Design review of the part shown in the three views and the two pictorial views. Dimensions are in mm from the part's minimum x, y and z. A direction names the side the tool comes from. Give positions to 0.01 mm unless a question says otherwise; leave off trailing zeros. Order: outer loops, then holes, each group sorted by start corner. A loop starts at its lowest first (then second) coordinate and runs counter-clockwise, first axis right, second up. Notation, with made-up numbers: (82, -36) - (113, -36) arc R13 cw to (113, -25) - close; hole circle Ø1 at (55.25, 84.25). An arc over 180 degrees is marked (long way). Put each result on its own line as item: value.
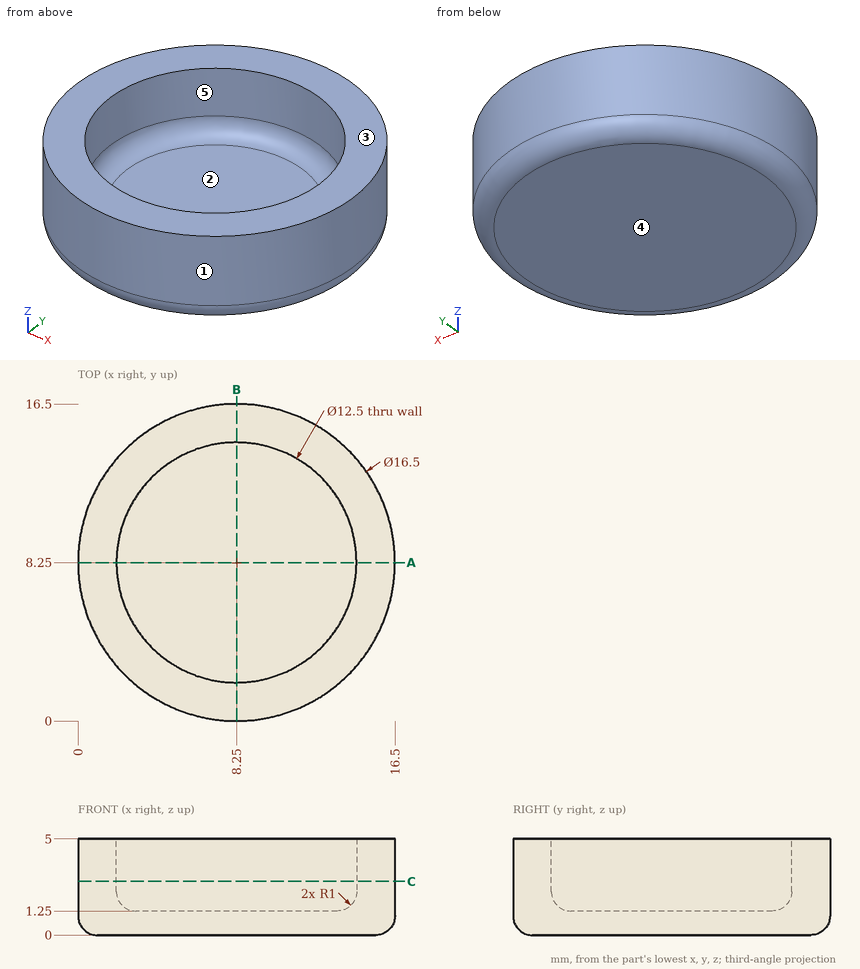
(1) The part is to be moulded in two halves that separate along Y. For the marked faces 1, 2 and 3, say which applies: pulls with the +Y half, pulls with the -Y half, needs draft (parallel to the pull), parting line crosses it, or undercut.
The answers:
face 1: parting line crosses it
face 2: undercut
face 3: needs draft
(2) For the marked faces 4 and 5, list the 3-axis set-ups (+Z, -Z, +X, -X, +Y, -Y) from which the entire face can be reached by the end or side of a thin tool; tool diameter is ignored.
The answers:
face 4: -Z, +X, -X, +Y, -Y
face 5: +Z
(3) Take a section at A-A, the plane y = 8.25. Write out the cut boundary in (x, z).
The answers:
outline: (0, 1) arc R1 ccw to (1, 0) - (15.5, 0) arc R1 ccw to (16.5, 1) - (16.5, 5) - (14.5, 5) - (14.5, 2.25) arc R1 cw to (13.5, 1.25) - (3, 1.25) arc R1 cw to (2, 2.25) - (2, 5) - (0, 5) - close
(4) Take a section at C-C, the plane z = 2.8. Write out the cut boundary in (x, y), then the cut area to 3 significant figures.
The answers:
outline: circle Ø16.5 at (8.25, 8.25); hole circle Ø12.5 at (8.25, 8.25)
area: 91.1 mm^2
(5) Clearance check with flat-ended pins moving along their axes: pin 1 Ø7.5 at (x, y) = (8.25, 8.25) entering from -Z; pin 2 Ø3 at (y, z) = (13, 3) entering from -X; pin 3 Ø1 at (x, y) = (8.5, 11) entering from +Z; pin 4 Ø1.5 at (y, z) = (2, 3) entering from -X. State where each tip first meets the part, or that it passes through.
The answers:
pin 1: z = 0
pin 2: x = 0.67
pin 3: z = 1.25
pin 4: x = 2.1
(6) Wall thickness on L1, parallel to Y at x = 8.25, z = 3.2; L2, parallel to X at y = 8.5, z = 2.3 (3 decimals); L3, parallel to Z at x = 8.75, y = 4.5: over which ranges is each line inside the solid? List them lowest first.
The answers:
L1: 0 to 2, 14.5 to 16.5
L2: 0.004 to 2.005, 14.495 to 16.496
L3: 0 to 1.25
